Could you check a few things on this model? Use its own coordinates, in mm. Face numbers are marked on the shaded views. Coordinates: 2 decimals unless noted, no trailing zeros. Order: outer loops, then holes, each group sorted by start corner. A loop starts at its lowest first (then second) coordinate and runs counter-clockwise, first axis right, second up. Notation, with made-up numbers: (-6, 81) -> (30, 81) arc R4 cw to (30, 87) -> close; hole circle Ø8 at (87, 22.25). An arc over 180 degrees is marked (long way). Put each result on its own line as item: value. Start each with the question number.
Q1. Please list where these lines run through material, in increasing order: line 1 along Y through (x, z) = (-9, 28.5); line 2 along Y through (x, z) = (30.5, 23); line 3 along Y through (x, z) = (-38, 22).
Q2. If we section it at A-A (x = 0): Please give me the cut outline in (y, z), and give its area (3 significant figures).
Q3. We'd pull the mould along Y, two halves only. Please class the marked faces 1, 2 and 3: +Y half, -Y half, draft (parallel to the pull), parting line (faces both ways), or undercut.
Q4. If we section it at B-B (y = 43.5): Please give me the cut outline in (x, z), and give its area (3 significant figures).
Q5. If we section it at C-C (z = 15.5): Please give me the cut outline in (x, y).
Q6. If we section it at D-D (y = -52): Please give me the cut outline in (x, z), and give its area (3 significant figures).
Q7. Will these pins go through, and if not, where does the flat tip stop? pin 1 (5 mm diameter, centred on x = 4.5, y = -1, fed in from +Z); pin 2 (8 mm diameter, centred on y = 27, z = -16, fed in from -X); pin 3 (3 mm diameter, centred on y = 16.5, z = -9, fed in from +X).
from build123d import *
from build123d import SkipClean  # not in build123d's __all__

# Parameters (mm, degrees)
F0_W     = 101.3660542667
F0_H     = 109.7881607711
F1_DEPTH = 69.596
F3_DEPTH = 101.3670542667
F5_DEPTH = 10.414
F7_DEPTH = 12.954
F8_R     = 15.6385789161
F9_DEPTH = 109.7891607711


# Not quite as in the source:
# - after a boolean that leaves OpenCascade's solid faulty, fix() repairs it


with BuildPart() as f1:
    # F0 (on Front) → F1 (new body, symmetric)
    with BuildSketch(Plane.XZ):
        with Locations((-2.2559221834, -7.3693413287)):
            Rectangle(F0_W, F0_H)
    extrude(amount=F1_DEPTH, both=True)

    # F2 (on face) → F3 (cut, through all)
    with BuildSketch(Plane.YZ.offset(48.42710495)):
        with BuildLine():
            Line((24.9655246735, 47.5247390568), (-24.0631587803, 47.5247390568))
            ThreePointArc((-24.0631587803, 47.5247390568), (0.4511829466, 18.0011880568), (24.9655246735, 47.5247390568))
        make_face()
    extrude(amount=-F3_DEPTH, mode=Mode.SUBTRACT)

    # F4 (on face) → F5 (join)
    with BuildSketch(Plane.YZ.offset(48.42710495)):
        with BuildLine():
            Line((-24.0631587803, 47.5247390568), (-32.028503716, 47.5247390568))
            ThreePointArc((-32.028503716, 47.5247390568), (0.372864306, 10.3342526114), (32.7742323279, 47.5247390568))
            Line((32.7742323279, 47.5247390568), (24.9655246735, 47.5247390568))
            ThreePointArc((24.9655246735, 47.5247390568), (0.4511829466, 18.0011880568), (-24.0631587803, 47.5247390568))
        make_face()
    with SkipClean():  # cleaning this boolean's faces spoils the solid; the shape is the same uncleaned
        extrude(amount=F5_DEPTH)

    # F6 (on face) → F7 (join)
    with BuildSketch(Plane(origin=(-52.9389493167, 0, 0), x_dir=(0, -1, 0), z_dir=(-1, 0, 0))):
        with BuildLine():
            Line((-24.9655246735, 47.5247390568), (-30.9813152999, 47.5247390568))
            ThreePointArc((-30.9813152999, 47.5247390568), (-0.1503955573, 12.1180891172), (30.6805241853, 47.5247390568))
            Line((30.6805241853, 47.5247390568), (24.0631587803, 47.5247390568))
            ThreePointArc((24.0631587803, 47.5247390568), (-0.4511829466, 18.0011880568), (-24.9655246735, 47.5247390568))
        make_face()
    extrude(amount=F7_DEPTH)

    add(f1.part.fix(), mode=Mode.REPLACE)

    # F8 (on face) → F9 (cut, through all)
    with BuildSketch(Plane.XY.offset(47.5247390568)):
        with Locations((0, 49.4834557176)):
            Circle(F8_R)
        with Locations((-2.8148e-06, -49.0286834538)):
            Circle(F8_R)
    extrude(amount=-F9_DEPTH, mode=Mode.SUBTRACT)


solid = f1.part
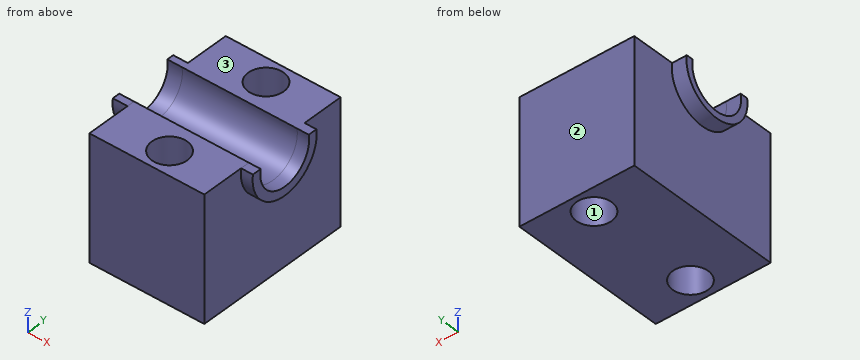
The answers:
1. line 1: -69.6 to -61.82, -36.24 to -19.88, 20.78 to 36.69, 62.27 to 69.6
1. line 2: -69.6 to -14.53, 15.43 to 69.6
1. line 3: -69.6 to -13.09, 14 to 69.6
2. outline: (-69.6, -62.26) -> (-64.67, -62.26) -> (-64.67, 47.52) -> (-69.6, 47.52) -> close; (-33.39, -62.26) -> (33.84, -62.26) -> (33.84, 47.52) -> (24.97, 47.52) arc R24.94 cw (long way) to (-24.06, 47.52) -> (-33.39, 47.52) -> close; (65.12, -62.26) -> (69.6, -62.26) -> (69.6, 47.52) -> (65.12, 47.52) -> close
2. area: 7,210 mm^2
3. face 1: undercut
3. face 2: +Y half
3. face 3: draft
4. outline: (-52.94, -62.26) -> (-14.45, -62.26) -> (-14.45, 47.52) -> (-52.94, 47.52) -> close; (14.45, -62.26) -> (48.43, -62.26) -> (48.43, 47.52) -> (14.45, 47.52) -> close
4. area: 7,960 mm^2
5. outline: (-65.89, -13.96) -> (-52.94, -13.96) -> (-52.94, -69.6) -> (48.43, -69.6) -> (48.43, -17.27) -> (58.84, -17.27) -> (58.84, 18.02) -> (48.43, 18.02) -> (48.43, 69.6) -> (-52.94, 69.6) -> (-52.94, 14.26) -> (-65.89, 14.26) -> close; hole circle Ø31.28 at (0, -49.03); hole circle Ø31.28 at (0, 49.48)
6. outline: (-52.94, -62.26) -> (-15.35, -62.26) -> (-15.35, 47.52) -> (-52.94, 47.52) -> close; (15.35, -62.26) -> (48.43, -62.26) -> (48.43, 47.52) -> (15.35, 47.52) -> close
6. area: 7,760 mm^2
7. pin 1: z = 18.32
7. pin 2: x = -52.94
7. pin 3: x = 48.43
